```python
from build123d import *

# Parameters (mm, degrees)
SKETCH1_R           = 28.25
SKETCH1_R_2         = 1.5
BOSS_EXTRUDE1_DEPTH = 3
FILLET1_R           = 25


with BuildPart() as part:
    # Sketch1 → Boss-Extrude1 (new body)
    with BuildSketch(Plane(origin=(0, 0, 0), x_dir=(1, 0, 0), z_dir=(0, 1, 0))):
        with BuildLine():
            ThreePointArc((-19.00522636, 26.055016235), (0, 32.25), (19.00522636, 26.055016235))
            ThreePointArc((19.00522636, 26.055016235), (26.339727599, 26.339727599), (26.055016235, 19.00522636))
            ThreePointArc((26.055016235, 19.00522636), (32.25, 0), (26.055016235, -19.00522636))
            ThreePointArc((26.055016235, -19.00522636), (26.339727599, -26.339727599), (19.00522636, -26.055016235))
            ThreePointArc((19.00522636, -26.055016235), (0, -32.25), (-19.00522636, -26.055016235))
            ThreePointArc((-19.00522636, -26.055016235), (-26.339727599, -26.339727599), (-26.055016235, -19.00522636))
            ThreePointArc((-26.055016235, -19.00522636), (-32.25, 0), (-26.055016235, 19.00522636))
            ThreePointArc((-26.055016235, 19.00522636), (-26.339727599, 26.339727599), (-19.00522636, 26.055016235))
        make_face()
        with Locations(Location((0, 0, 0), (0, 0, 270))):
            Circle(SKETCH1_R, mode=Mode.SUBTRACT)
        with Locations(Location((23.511300474, 23.511300474, 0), (0, 0, 270))):
            Circle(SKETCH1_R_2, mode=Mode.SUBTRACT)
        with Locations(Location((23.511300474, -23.511300474, 0), (0, 0, 270))):
            Circle(SKETCH1_R_2, mode=Mode.SUBTRACT)
        with Locations(Location((-23.511300474, -23.511300474, 0), (0, 0, 270))):
            Circle(SKETCH1_R_2, mode=Mode.SUBTRACT)
        with Locations(Location((-23.511300474, 23.511300474, 0), (0, 0, 270))):
            Circle(SKETCH1_R_2, mode=Mode.SUBTRACT)
    extrude(amount=BOSS_EXTRUDE1_DEPTH)

    # Fillet1
    fillet1_edges = [part.edges().sort_by_distance(p)[0] for p in [
        (-19.00522636, 1.5, -26.055016235),
        (19.00522636, 1.5, -26.055016235),
        (26.055016235, 1.5, -19.00522636),
        (26.055016235, 1.5, 19.00522636),
        (19.00522636, 1.5, 26.055016235),
        (-19.00522636, 1.5, 26.055016235),
        (-26.055016235, 1.5, 19.00522636),
        (-26.055016235, 1.5, -19.00522636),
    ]]
    fillet(fillet1_edges, radius=FILLET1_R)


solid = part.part
```
Work out the finished part from the listing and answer in its coordinate system (mm). Give positions to 0.01 mm unless a question says otherwise; leave off trailing zeros. Order: outer loops, then holes, each group sorted by start corner. A loop starts at its lowest first (then second) coordinate and runs counter-clockwise, first axis right, second up. Notation, with made-up numbers: (-9, -8) - (0, -8) arc R26 ccw to (0, 28) - close; hole circle Ø8 at (24, -32). An arc over 180 degrees is marked (long way). One line per item, written item: value. Start each with the question number.
1. Section C-C, the plane y = 0.9 is taken. Count the separate pieces of the cut face and the enclosed holes in it, then the cut area to 3 significant figures.
2. Section A-A, the plane x = 0 is taken. Write down the section's boundary in (y, z), then the cut area to 3 significant figures.
3. This flat-tipped pin is pushed along its axis until it touches: pin 1 Ø1 at (x, y) = (0, 2.5) entering from +Z. Where does it stop, or does it pass through?
4. Section B-B, the plane z = 0 is taken. Write down the section's boundary in (x, y).
5. Consider line 1 (Z direction, x = 24, y = 1.65); line 2 (Z direction, x = -9, y = 1.55); line 3 (Z direction, x = 10.5, y = 0.4). Determine where each line is inside the solid, lowest interval first.
6. For a pull along X with two mould halves and no side action, classify faces 1 (the face through (22.937, 1.479, -22.126)), 2 (the face through (-24.086, 1.479, -22.126)), 3 (the face through (-32.25, 1.48, 0.18)), 4 (the face through (-0.18, 1.48, -32.25)) as released by +X, released by -X, zero draft, split by the parting line, or undercut.
Filled sheet:
1. separate pieces: 1
1. enclosed holes: 5
1. area: 946 mm²
2. outline: (0, -32.25) - (3, -32.25) - (3, -28.25) - (0, -28.25) - close; (0, 28.25) - (3, 28.25) - (3, 32.25) - (0, 32.25) - close
2. area: 24.0 mm²
3. pin 1: z = 32.25
4. outline: (-32.25, 0) - (-28.25, 0) - (-28.25, 3) - (-32.25, 3) - close; (28.25, 0) - (32.25, 0) - (32.25, 3) - (28.25, 3) - close
5. line 1: -27.66 to -24.93, -22.09 to -14.9, 14.9 to 22.09, 24.93 to 27.66
5. line 2: -30.97 to -26.78, 26.78 to 30.97
5. line 3: -30.49 to -26.23, 26.23 to 30.49
6. face 1: undercut
6. face 2: undercut
6. face 3: released by -X
6. face 4: split by the parting line
